from build123d import *

# Parameters (mm, degrees)
SKETCH1_W           = 360
SKETCH1_H           = 283
SKETCH1_R           = 2.2
SKETCH1_R_2         = 2.25
BOSS_EXTRUDE1_DEPTH = 1
SKETCH3_R           = 18.999999993
SKETCH3_R_2         = 1.499999993
SKETCH3_W           = 1
SKETCH3_H           = 283
CUT_EXTRUDE1_DEPTH  = 1
SKETCH4_W           = 360
SKETCH4_H           = 6
BOSS_EXTRUDE2_DEPTH = 1


with BuildPart() as part:
    # Sketch1 → Boss-Extrude1 (new body)
    with BuildSketch(Plane(origin=(0, 0, 0), x_dir=(0, 0, -1), z_dir=(1, 0, 0))):
        Rectangle(SKETCH1_W, SKETCH1_H)
        with Locations((-167, 123.5)):
            Circle(SKETCH1_R, mode=Mode.SUBTRACT)
        with Locations((-167, -129.5)):
            Circle(SKETCH1_R, mode=Mode.SUBTRACT)
        with Locations(Location((161, 123.5, 0), (0, 0, 180))):
            Circle(SKETCH1_R, mode=Mode.SUBTRACT)
        with Locations(Location((161, -129.5, 0), (0, 0, 180))):
            Circle(SKETCH1_R, mode=Mode.SUBTRACT)
        with Locations((-166.5, 97.000820447)):
            Circle(SKETCH1_R_2, mode=Mode.SUBTRACT)
        with Locations((-166.5, 77.000820447)):
            Circle(SKETCH1_R_2, mode=Mode.SUBTRACT)
        with Locations((-166.5, -82.999179553)):
            Circle(SKETCH1_R_2, mode=Mode.SUBTRACT)
        with Locations((-166.5, -102.999179553)):
            Circle(SKETCH1_R_2, mode=Mode.SUBTRACT)
    extrude(amount=BOSS_EXTRUDE1_DEPTH)

    # Sketch3 → Cut-Extrude1 (cut)
    with BuildSketch(Plane(origin=(1, 0, 0), x_dir=(0, 0, -1), z_dir=(1, 0, 0))):
        with Locations((-90.763094033, -96.299179553)):
            Circle(SKETCH3_R)
        with Locations((-106.763094033, -80.299179553)):
            Circle(SKETCH3_R_2)
        with Locations((-74.763094033, -80.299179553)):
            Circle(SKETCH3_R_2)
        with Locations((-74.763094033, -112.299179553)):
            Circle(SKETCH3_R_2)
        with Locations((-106.763094033, -112.299179553)):
            Circle(SKETCH3_R_2)
        with Locations((-179.5, 0)):
            Rectangle(SKETCH3_W, SKETCH3_H)
    extrude(amount=-CUT_EXTRUDE1_DEPTH, mode=Mode.SUBTRACT)

    # Sketch4 → Boss-Extrude2 (add)
    with BuildSketch(Plane.ZY):
        with Locations((0, -144.5)):
            Rectangle(SKETCH4_W, SKETCH4_H)
    extrude(amount=-BOSS_EXTRUDE2_DEPTH)


solid = part.part
Read the model definition and answer for the solid it produces. Units are mm, in the model's axes. Round coordinates to 2 decimals unless told otherwise and drop trailing zeros.
1) The part is cut by section A-A on x = 0.3. Give the number of separate pieces and of enclosed holes in the cut face, plus the area to 3 significant figures.
2) The mould has two halves that part along Y. Classify faces 1 (the face through (0, -1, -3)), 2 (the face through (0.51, -83.46, 104.77)): released by +Y, released by -Y, zero draft, split by the parting line, or undercut.
3) Straight lines are drawn through the part: L1, parallel to Y at x = 0.6, z = -161; L2, parallel to Y at x = 0.35, z = -163; L3, parallel to Z at x = 0.6, y = 3. For each, find the intervals that lie inside material, in ascending order.
Resolved:
1. separate pieces: 1
1. enclosed holes: 13
1. area: 102,000 mm2
2. face 1: zero draft
2. face 2: undercut
3. L1: y = -147.5 to -131.7, -127.3 to 121.3, 125.7 to 141.5
3. L2: y = -147.5 to -130.42, -128.58 to 122.58, 124.42 to 141.5
3. L3: z = -180 to 179
